```python
from build123d import *

# Parameters (mm, degrees)
SKETCH1_R           = 2.75
BOSS_EXTRUDE1_DEPTH = 3
SKETCH2_R           = 1.5
BOSS_EXTRUDE2_DEPTH = 10
CUT_EXTRUDE1_DEPTH  = 1.5


with BuildPart() as part:
    # Sketch1 → Boss-Extrude1 (new body)
    with BuildSketch(Plane(origin=(0, 0, 0), x_dir=(1, 0, 0), z_dir=(0, 1, 0))):
        Circle(SKETCH1_R)
    extrude(amount=BOSS_EXTRUDE1_DEPTH)

    # Sketch2 → Boss-Extrude2 (add)
    with BuildSketch(Plane(origin=(0, 3, 0), x_dir=(1, 0, 0), z_dir=(0, 1, 0))):
        Circle(SKETCH2_R)
    extrude(amount=BOSS_EXTRUDE2_DEPTH)

    # Sketch3 → Cut-Extrude1 (cut)
    with BuildSketch(Plane(origin=(0, 0, 0), x_dir=(-1, 0, 0), z_dir=(0, -1, 0))):
        Polygon((0, -1.443375673), (1.25, -0.721687836), (1.25, 0.721687836), (0, 1.443375673), (-1.25, 0.721687836), (-1.25, -0.721687836), align=None)
    extrude(amount=-CUT_EXTRUDE1_DEPTH, mode=Mode.SUBTRACT)


solid = part.part
```
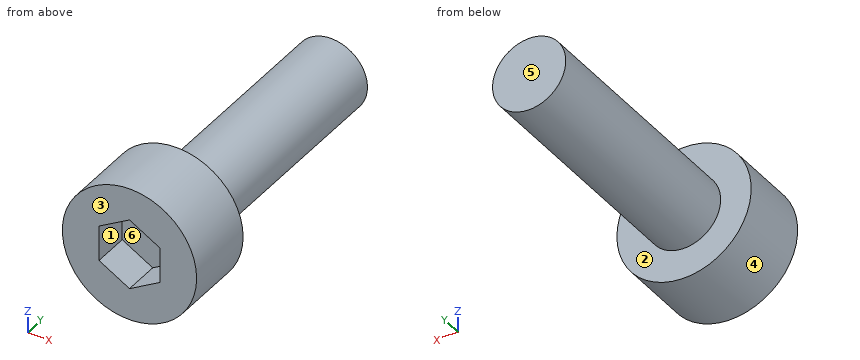
Part model, mm, in its own coordinate system. Face numbers are marked on the shaded views. A direction names the side the tool comes from. Round coordinates to 2 decimals unless told otherwise and drop trailing zeros. Loops run counter-clockwise (first coordinate to the right, second up) from the corner with the lowest first, then second, coordinate; pieces in that order, holes last. Notation, with made-up numbers: (65.25, 23) -> (107.25, 23) arc R35 ccw to (107.25, 62) -> close; hole circle Ø7 at (56.5, 55.5). An arc over 180 degrees is marked (long way). Use one line per item in the form item = value. Start each with the question number.
Item 1: Drill centre lines: line 1 along Y through (x, z) = (-0.6, 2.55); line 2 along Y through (x, z) = (0.8, 0.7); line 3 along X through (y, z) = (6.25, 0.4). Where is each one in solid material? Low to high.
Item 2: Band-saw the part on C-C (y = 5.75). List the corners of the cut face in (x, z).
Item 3: Tool access for the marked faces 1, 2 and 3: list every direction of +Z, -Z, +X, -X, +Y, -Y with a clear straight run to the whole face (end or side of a thin tool).
Item 4: Band-saw the part on D-D (x = -2.4). List the corners of the cut face in (y, z).
Item 5: Band-saw the part on A-A (z = 0). List the corners of the cut face in (x, y), plus the area to 4 significant figures.
Item 6: Drop flat-ended pins along their axis: pin 1 Ø1.6 at (y, z) = (0.5, 0.5) entering from -X; pin 2 Ø3 at (x, y) = (-2, 5) entering from -Z; pin 3 Ø2 at (y, z) = (7, 0) entering from +X; pin 4 Ø1.5 at (y, z) = (6, 1.5) entering from +X. Give the stop position or say it passes through.
Item 7: Band-saw the part on B-B (x = -0.9). List the corners of the cut face in (y, z), plus the area to 3 significant figures.
Item 8: Two-plate mould, pull along X, no slides. Class the marked faces 4, 5 and 6: released by +X, released by -X, zero draft, split by the parting line, or undercut.
Data:
q1.line_1 = 0 to 3
q1.line_2 = 1.5 to 13
q1.line_3 = -1.45 to 1.45
q2.outline = circle Ø3 at (0, 0)
q3.face_1 = -Y
q3.face_2 = +Y
q3.face_3 = +Z, -Z, +X, -X, -Y
q4.outline = (0, -1.34) -> (3, -1.34) -> (3, 1.34) -> (0, 1.34) -> close
q5.outline = (-2.75, 0) -> (-1.25, 0) -> (-1.25, 1.5) -> (1.25, 1.5) -> (1.25, 0) -> (2.75, 0) -> (2.75, 3) -> (1.5, 3) -> (1.5, 13) -> (-1.5, 13) -> (-1.5, 3) -> (-2.75, 3) -> close
q5.area = 42.75 mm^2
q6.pin_1 = -2.75
q6.pin_2 = -1.41
q6.pin_3 = 1.5
q6.pin_4 = 1.3
q7.outline = (0, -2.6) -> (3, -2.6) -> (3, -1.2) -> (13, -1.2) -> (13, 1.2) -> (3, 1.2) -> (3, 2.6) -> (0, 2.6) -> (0, 0.92) -> (1.5, 0.92) -> (1.5, -0.92) -> (0, -0.92) -> close
q7.area = 36.8 mm^2
q8.face_4 = split by the parting line
q8.face_5 = zero draft
q8.face_6 = undercut
